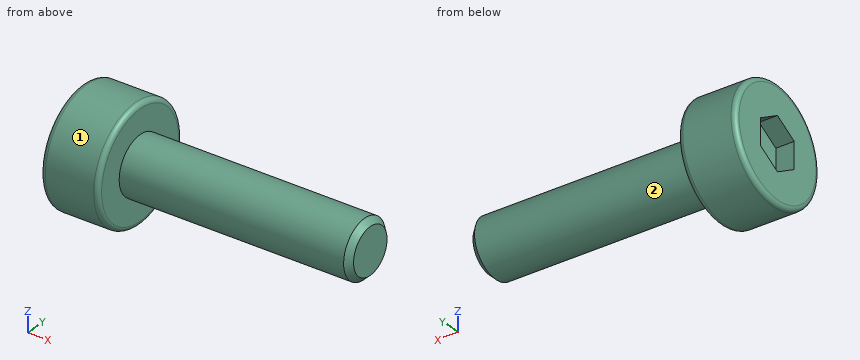
```python
from build123d import *

# Parameters (mm, degrees)
CUT_EXTRUDE1_DEPTH = 0.8


with BuildPart() as part:
    # Sketch2 → Revolve1 (revolve)
    with BuildSketch(Plane.XY, mode=Mode.PRIVATE) as revolve1_sk:
        with BuildLine():
            Line((0, 0), (0, 2.3))
            ThreePointArc((0, 2.3), (0.058578644, 2.441421356), (0.2, 2.5))
            Line((0.2, 2.5), (2.3, 2.5))
            ThreePointArc((2.3, 2.5), (2.441421356, 2.441421356), (2.5, 2.3))
            Line((2.5, 2.3), (2.5, 1.25))
            Line((2.5, 1.25), (12.25, 1.25))
            Line((12.25, 1.25), (12.5, 1))
            Line((12.5, 1), (12.5, 0))
            Line((12.5, 0), (0, 0))
        make_face()
    revolve(revolve1_sk.sketch.rotate(Axis((-2.281841559, 0, 0), (1, 0, 0)), 90), axis=Axis((-2.281841559, 0, 0), (1, 0, 0)))

    # Sketch3 → Cut-Extrude1 (cut)
    with BuildSketch(Plane.ZY):
        Polygon((0.577350269, -1), (1.154700538, 0), (0.577350269, 1), (-0.577350269, 1), (-1.154700538, 0), (-0.577350269, -1), align=None)
    extrude(amount=-CUT_EXTRUDE1_DEPTH, mode=Mode.SUBTRACT)


solid = part.part
```
The listing builds one solid part. Answer for the finished solid, in the listing's coordinates (mm). Face numbers are marked on the shaded views. A direction names the side the tool comes from. Give positions to 0.01 mm unless a question says otherwise; leave off trailing zeros. Order: outer loops, then holes, each group sorted by start corner. A loop starts at its lowest first (then second) coordinate and runs counter-clockwise, first axis right, second up. Notation, with made-up numbers: M 17.25,-29 L 74.25,-29 A34 ccw 74.25,10 Z; hole C -5.5,-8 d6. An arc over 180 degrees is marked long. Put each result on its own line as item: value. Start each with the question number.
Item 1: Find the intervals of material crossed by line 1 along X through (y, z) = (-0.55, 0.8); line 2 along X through (y, z) = (2, 0); line 3 along Y through (x, z) = (0.5, 0.2), in increasing order.
Item 2: A flat-ended cylindrical pin translates along its axis: P1, Ø2, axis at y = 0, z = -0.5, coming from the -X side. Find the tip coordinate at first contact, or state that the pin passes through.
Item 3: The part is cut by section A-A, the plane z = 0. Determine the outline of the cut face in (x, y).
Item 4: Which of the six approach directions +Z, -Z, +X, -X, +Y, -Y give full straight-line access (tool end or side, diameter ignored) to the marked faces 1 and 2?
Item 5: The part is cut by section B-B, the plane x = 10.25. Determine the outline of the cut face in (y, z), and give its area (3 significant figures).
Answer key:
1. line 1: x = 0.8 to 12.5
1. line 2: x = 0 to 2.5
1. line 3: y = -2.49 to -1, 1 to 2.49
2. P1: stops at x = 0
3. outline: M 0,-2.3 A0.2 ccw 0.2,-2.5 L 2.3,-2.5 A0.2 ccw 2.5,-2.3 L 2.5,-1.25 L 12.25,-1.25 L 12.5,-1 L 12.5,1 L 12.25,1.25 L 2.5,1.25 L 2.5,2.3 A0.2 ccw 2.3,2.5 L 0.2,2.5 A0.2 ccw 0,2.3 L 0,1 L 0.8,1 L 0.8,-1 L 0,-1 Z
4. face 1: +X, -X
4. face 2: +X
5. outline: C 0,0 d2.5
5. area: 4.91 mm²
